For this review, take the finished solid that the model builds, in its own axes (mm). A direction names the side the tool comes from. Coordinates: 2 decimals unless noted, no trailing zeros. Loops run counter-clockwise (first coordinate to the right, second up) from the corner with the lowest first, then second, coordinate; pieces in that order, holes last. Notation, with made-up numbers: M -31.75,34 L -21.75,34 A27 ccw -21.75,61 Z; hole C 88.5,46.5 d2. An arc over 180 degrees is marked long. Answer as a JSON object with one key per item and string values. Group by question number.
Item 1: Add section D-D (x = -3.5). State the section outline as (y, z) points, then the cut area to 3 significant figures.
Item 2: Wall thickness on L1, parallel to X at y = 6.25, z = 5.25; L2, parallel to Y at x = -7.6, z = 3; L3, parallel to X at y = 14, z = 0.4: over which ranges is each line inside the solid? List them lowest first. Write a range as from..to.
Item 3: Insertion check: pin 1 (3 mm diameter, centred on y = 5, z = 4, fed in from +X); pin 2 (1.8 mm diameter, centred on y = 3, z = 3, fed in from +X); pin 3 (2 mm diameter, centred on x = -4.5, z = 3.5, fed in from +Y); pin 4 (3 mm diameter, centred on x = -7, z = 0.5, fed in from +Y). Each pin has a flat end and moves straight along its axis. Give the tip position at first contact, or say it passes through.
Item 4: Tool access review of faces 5 (the face through (-5, 11, 0)), 6 (the face through (-5, 8, 3)), 7 (the face through (-2, 0, 3)), 8 (the face through (-5, 13, 3)), 9 (the face through (-7, 16, 3)): name each direction out of +Z, -Z, +X, -X, +Y, -Y from which nothing blocks a thin tool from reaching the whole face with its end or side.
Item 5: Add section B-B (y = 14). State the section outline as (x, z) points.
Item 6: Add section C-C (y = 3.5). State the section outline as (x, z) points.
Item 7: Mouldability with a two-part tool opening along X and no side actions: class faces 1 (the face through (-10, 10, 3)), 2 (the face through (-6.25, 5, 3)), 3 (the face through (-5, 19, 3.1)), 4 (the face through (-9, 21, 3)) as +X half, -X half, draft (parallel to the pull), parting line (faces both ways), or undercut.
Item 8: Add section A-A (z = 3.7). State the section outline as (x, y) points.
from build123d import *

# Parameters (mm, degrees)
SALIENTE_EXTRUIR1_DEPTH = 6
REDONDEO1_RADIUS        = 3
REDONDEO1_LENGTH        = 3.75
REDONDEO2_RADIUS        = 3
REDONDEO2_LENGTH        = 3
REDONDEO3_RADIUS        = 3
REDONDEO3_LENGTH        = 3
REDONDEO4_RADIUS        = 3
REDONDEO4_LENGTH        = 3.75
CORTAR_EXTRUIR1_REACH   = 26.021
CROQUIS2_R              = 1.5
SALIENTE_EXTRUIR3_REACH = 24.935
CROQUIS4_R              = 1


with BuildPart() as part:
    # Croquis1 → Saliente-Extruir1 (new body)
    with BuildSketch(Plane.XY):
        Polygon((-7, 21), (-7, 13), (-3, 13), (-3, 21), (0, 21), (0, 0), (-3.75, 0), (-3.75, 8), (-6.25, 8), (-6.25, 0), (-10, 0), (-10, 21), align=None)
    extrude(amount=SALIENTE_EXTRUIR1_DEPTH)

    # Redondeo1: full round fillet: the end face becomes a half cylinder, R = half its width
    redondeo1_face = Plane((-1.875, 0, 3), x_dir=(1, 0, 0), z_dir=(0, -1, 0))  # on the end face: x along it, z out of the body
    redondeo1_slab = redondeo1_face.offset(-REDONDEO1_RADIUS / 2) * Box(REDONDEO1_LENGTH, 2 * REDONDEO1_RADIUS, REDONDEO1_RADIUS, mode=Mode.PRIVATE)  # the body's end, R deep
    redondeo1_round = Plane((-1.875, 3, 3), x_dir=(0, -1, 0), z_dir=(1, 0, 0)) * Cylinder(REDONDEO1_RADIUS, REDONDEO1_LENGTH, mode=Mode.PRIVATE)  # its axis R under the face
    add(redondeo1_slab - redondeo1_round, mode=Mode.SUBTRACT)

    # Redondeo2: full round fillet: the end face becomes a half cylinder, R = half its width
    redondeo2_face = Plane((-1.5, 21, 3), x_dir=(-1, 0, 0), z_dir=(0, 1, 0))  # on the end face: x along it, z out of the body
    redondeo2_slab = redondeo2_face.offset(-REDONDEO2_RADIUS / 2) * Box(REDONDEO2_LENGTH, 2 * REDONDEO2_RADIUS, REDONDEO2_RADIUS, mode=Mode.PRIVATE)  # the body's end, R deep
    redondeo2_round = Plane((-1.5, 18, 3), x_dir=(0, 1, 0), z_dir=(-1, 0, 0)) * Cylinder(REDONDEO2_RADIUS, REDONDEO2_LENGTH, mode=Mode.PRIVATE)  # its axis R under the face
    add(redondeo2_slab - redondeo2_round, mode=Mode.SUBTRACT)

    # Redondeo3: full round fillet: the end face becomes a half cylinder, R = half its width
    redondeo3_face = Plane((-8.5, 21, 3), x_dir=(-1, 0, 0), z_dir=(0, 1, 0))  # on the end face: x along it, z out of the body
    redondeo3_slab = redondeo3_face.offset(-REDONDEO3_RADIUS / 2) * Box(REDONDEO3_LENGTH, 2 * REDONDEO3_RADIUS, REDONDEO3_RADIUS, mode=Mode.PRIVATE)  # the body's end, R deep
    redondeo3_round = Plane((-8.5, 18, 3), x_dir=(0, 1, 0), z_dir=(-1, 0, 0)) * Cylinder(REDONDEO3_RADIUS, REDONDEO3_LENGTH, mode=Mode.PRIVATE)  # its axis R under the face
    add(redondeo3_slab - redondeo3_round, mode=Mode.SUBTRACT)

    # Redondeo4: full round fillet: the end face becomes a half cylinder, R = half its width
    redondeo4_face = Plane((-8.125, 0, 3), x_dir=(1, 0, 0), z_dir=(0, -1, 0))  # on the end face: x along it, z out of the body
    redondeo4_slab = redondeo4_face.offset(-REDONDEO4_RADIUS / 2) * Box(REDONDEO4_LENGTH, 2 * REDONDEO4_RADIUS, REDONDEO4_RADIUS, mode=Mode.PRIVATE)  # the body's end, R deep
    redondeo4_round = Plane((-8.125, 3, 3), x_dir=(0, -1, 0), z_dir=(1, 0, 0)) * Cylinder(REDONDEO4_RADIUS, REDONDEO4_LENGTH, mode=Mode.PRIVATE)  # its axis R under the face
    add(redondeo4_slab - redondeo4_round, mode=Mode.SUBTRACT)

    # Cortar-Extruir1: up to this face of the body (flat: up to its plane)
    cortar_extruir1_end = Plane(part.part.faces().sort_by_distance((-10, 10.5, 3))[0])
    # Croquis2 → Cortar-Extruir1 (cut, up to the picked face)
    with BuildSketch(Plane(origin=(0, 0, 0), x_dir=(0, 0, -1), z_dir=(1, 0, 0)), mode=Mode.PRIVATE) as cortar_extruir1_sk1:
        with Locations((-3, 3)):
            Circle(CROQUIS2_R)
    cortar_extruir1_tool1 = split(extrude(cortar_extruir1_sk1.sketch, amount=-CORTAR_EXTRUIR1_REACH, mode=Mode.PRIVATE), bisect_by=cortar_extruir1_end, keep=Keep.BOTH, mode=Mode.PRIVATE)
    add(cortar_extruir1_tool1.solids().sort_by(Axis((0, 3, 3), (-1, 0, 0)))[0], mode=Mode.SUBTRACT)

    # Croquis4 → Saliente-Extruir3 (add, up to next)
    with BuildSketch(Plane(origin=(-7, 0, 0), x_dir=(0, 0, -1), z_dir=(1, 0, 0)), mode=Mode.PRIVATE) as saliente_extruir3_sk1:
        with Locations(Location((-3.130856321, 18, 0), (0, 0, 270))):
            Circle(CROQUIS4_R)
    saliente_extruir3_tool1 = extrude(saliente_extruir3_sk1.sketch, amount=SALIENTE_EXTRUIR3_REACH, mode=Mode.PRIVATE) - part.part
    add(saliente_extruir3_tool1.solids().sort_by_distance((-7, 18, 3.130856))[0])


solid = part.part
From the geometry:
{
 "1": {"outline": "M 3,0 L 13,0 L 13,6 L 3,6 A3 ccw Z; C 18,3.13 d2; hole C 3,3 d3", "area": "70.2 mm²"},
 "2": {"L1": "x = -10..-6.25, -3.75..0", "L2": "y = 0..1.5, 4.5..21", "L3": "x = -10..-7, -3..0"},
 "3": {"pin 1": "stops at x = 0", "pin 2": "passes through", "pin 3": "stops at y = 19", "pin 4": "stops at y = 20.83"},
 "4": {"face 5": "-Z, +X, -X, +Y, -Y", "face 6": "+Z, -Z, -Y", "face 7": "+X, -X, -Y", "face 8": "+Z, -Z", "face 9": "none"},
 "5": {"outline": "M -10,0 L -7,0 L -7,6 L -10,6 Z; M -3,0 L 0,0 L 0,6 L -3,6 Z"},
 "6": {"outline": "M -10,0 L -6.25,0 L -6.25,1.59 L -10,1.59 Z; M -10,4.41 L -6.25,4.41 L -6.25,6 L -10,6 Z; M -3.75,0 L 0,0 L 0,1.59 L -3.75,1.59 Z; M -3.75,4.41 L 0,4.41 L 0,6 L -3.75,6 Z"},
 "7": {"face 1": "-X half", "face 2": "undercut", "face 3": "undercut", "face 4": "draft"},
 "8": {"outline": "M -10,0.08 L -6.25,0.08 L -6.25,1.67 L -10,1.67 Z; M -10,4.33 L -6.25,4.33 L -6.25,8 L -3.75,8 L -3.75,4.33 L 0,4.33 L 0,20.92 L -3,20.92 L -3,18.82 L -7,18.82 L -7,20.92 L -10,20.92 Z; M -3.75,0.08 L 0,0.08 L 0,1.67 L -3.75,1.67 Z; hole M -7,13 L -3,13 L -3,17.18 L -7,17.18 Z"}
}
